Autodesk Inventor part; units mm, degrees
ref_plane "Start Plane" through (0, 0, -2.9702) normal (0, 0, 1) x (1, 0, 0)
ref_plane "End Plane" through (0, 0, 105) normal (0, 0, 1) x (1, 0, 0)
ref_plane "Work Plane4" through (0, -10, -2.9702) normal (0, 0.2847, -0.9586) x (1, 0, 0)
ref_plane "Start Plane" through (0, 0, -2.9702) normal (0, 0, 1) x (1, 0, 0)
ref_plane "End Plane" through (0, 0, 105) normal (0, 0, 1) x (1, 0, 0)
sketch "Sketch" plane through (0, 0, 0) normal (0, 0, 1) x (1, 0, 0)
  line L0 (-10, -7) -> (-10, 7)
  line L1 (-7, 10) -> (7, 10)
  line L2 (10, 7) -> (10, -7)
  line L3 (7, -10) -> (-7, -10)
  arc A0 (-10, -7) -> (-7, -10) centre (-7, -7) ccw
  arc A1 (-7, 10) -> (-10, 7) centre (-7, 7) ccw
  arc A2 (10, 7) -> (7, 10) centre (7, 7) ccw
  arc A3 (7, -10) -> (10, -7) centre (7, -7) ccw
  arc A4 (-7, 8) -> (-8, 7) centre (-7, 7) ccw
  line L4 (-7, 8) -> (7, 8)
  arc A5 (8, 7) -> (7, 8) centre (7, 7) ccw
  line L5 (8, 7) -> (8, -7)
  arc A6 (7, -8) -> (8, -7) centre (7, -7) ccw
  line L6 (7, -8) -> (-7, -8)
  arc A7 (-8, -7) -> (-7, -8) centre (-7, -7) ccw
  line L7 (-8, -7) -> (-8, 7)
  line L8 (0, 14.8698) -> (0, -14.8698) construction
  line L9 (-14.8698, 0) -> (14.8698, 0) construction
  dimension "d7" = 3
  dimension "d10" = 20
  dimension "d11" = 20
  dimension "d12" = 2
  dimension "d15" = 10
  dimension "d16" = 10
extrude "Body" add sketch "Sketch" along normal up to surface (107.9702 mm away) from surface at -2.9702
sketch "Sketch3" plane through (0, 0, 0) normal (0, 0, 1) x (1, 0, 0)
  line L0 (0, 0) -> (10, 0)
ref_plane "Work Plane3" through (0, 0, 0) normal (0, -1, 0) x (1, 0, 0)
sketch "Sketch4" plane through (0, 0, 0) normal (0, -1, 0) x (1, 0, 0)
  line L0 (-2, -2.9702) -> (12, -2.9702)
  line L1 (-2, 105) -> (12, 105)
  dimension "d18" = 107.9702
ref_plane "Work Plane4" through (0, -10, -2.9702) normal (0, 0.2847, -0.9586) x (1, 0, 0)
split "Split1" plane through (0, -10, -2.9702) removes the side toward (0, 0.2847, -0.9586)
sketch "Sketch5" plane through (-7, -10, 105) normal (0, -1, 0) x (1, 0, 0)
  line L0 (0, 0) -> (14, 0)
  line L1 (7, 0) -> (7, -18) construction
  line L2 (13.85, 0) -> (0.15, 0)
  line L3 (0.15, 0) -> (0.15, -18)
  line L4 (0.15, -18) -> (13.85, -18)
  line L5 (13.85, -18) -> (13.85, 0)
  line L6 (14, 0) -> (0, 0)
  line L7 (13.85, -8) -> (0.15, -8)
  line L8 (0.15, -8) -> (0.15, -26)
  line L9 (0.15, -26) -> (13.85, -26)
  line L10 (13.85, -26) -> (13.85, -8)
  line L11 (13.85, -8) -> (0.15, -26) construction
  line L12 (0.15, -8) -> (13.85, -26) construction
  line L13 (13.85, -8) -> (17, -8)
  line L14 (17, 0) -> (17, -102.9209)
  line L15 (17, -8) -> (17, 0)
  line L16 (17, 0) -> (13.85, 0)
  line L17 (-3, 0) -> (0, 0)
  line L18 (0.15, 0) -> (-3, 0)
  line L19 (-3, 0) -> (-3, -8)
  line L20 (-3, -8) -> (0.15, -8)
  point P0 (7, -105)
  point P1 (7, 0)
  point P2 (13.85, 0)
  point P3 (0.15, 0)
  point P4 (7, -17)
  point P5 (13.85, -18)
  point P6 (0.15, -18)
  point P7 (13.85, -8)
  point P8 (17, -8)
  point P9 (0.15, -8)
  dimension "d19" = 13.7
  dimension "d20" = 18
  dimension "d23" = 13.7
  dimension "d24" = 18
  dimension "d25" = 8
extrude "Extrusion2" cut sketch "Sketch5" against normal through all
equation "\"d7\" = G_IR"
equation "\"d10\" = G_H"
equation "\"d11\" = G_W"
equation "\"d12\" = G_T"
equation "\"d15\" = 0.5 * d10"
equation "\"d16\" = 0.5 * d11"
equation "\"d3\" = G_L"
equation "\"d23\" = d19"
equation "\"d24\" = d20"
equation "\"G_W\" = 20"
equation "\"G_H\" = 20"
equation "\"G_T\" = 2"
equation "\"G_IR\" = 3"
equation "\"G_L\" = d18"
equation "\"G_OFFSET_START\" = 2.97016"
equation "\"G_OFFSET_END\" = 0"
equation "\"d13\" = -G_OFFSET_START"
equation "\"d14\" = G_OFFSET_END + B_L"
equation "\"B_L\" = 105"
properties part number "ISO 12633-2 - 20x20x2 - 107,97" material "Steel, Mild"
Work out the finished part from the listing and answer in its coordinate system (mm). A direction names the side the tool comes from. Round coordinates to 2 decimals unless told otherwise and drop trailing zeros. Order: outer loops, then holes, each group sorted by start corner. A loop starts at its lowest first (then second) coordinate and runs counter-clockwise, first axis right, second up.
Q1. Given pin 1 Ø0.6 at (x, y) = (-2.5, -9.5) entering from +Z; pin 2 Ø12 at (x, y) = (-7, -6) entering from +Z; pin 3 Ø0.6 at (y, z) = (9, 89) entering from -X; pin 4 Ø1 at (y, z) = (9.5, 91.5) entering from +X, each flat-ended and moving along its own axis, determine where each tip first touches the part or whether it passes through.
Solution:
pin 1: stops at z = 79
pin 2: stops at z = 97
pin 3: stops at x = -9.47
pin 4: stops at x = 9.24
Q2. A tool of negligible diameter and unlimited length cuts with its end or side. For faces 1 (the flat face through (0, -8, 36)), 2 (the flat face through (-6.85, -9, 88)), 3 (the flat face through (0, -10, 35)), from which of +Z, -Z, +X, -X, +Y, -Y can it reach the whole face along a straight path? Write none if from no direction.
Solution:
face 1: +Z, -Z
face 2: +Z, +Y, -Y
face 3: +Z, -Z, +X, -X, -Y
Q3. Find the intervals of material crossed by line 1 along Y through (x, z) = (-3.25, 74); line 2 along X through (y, z) = (-7.5, 40), in increasing order.
Solution:
line 1: y = -10 to -8, 8 to 10
line 2: x = -9.96 to -7.87, 7.87 to 9.96
Q4. A cutting plane is placed at B-B, the plane z = 87. Determine the outline of the cut face in (x, y), then the cut area to 3 significant figures.
Solution:
outline: (-10, -7) arc R3 ccw to (-7, -10) - (-6.85, -10) - (-6.85, -8) - (-7, -8) arc R1 cw to (-8, -7) - (-8, 7) arc R1 cw to (-7, 8) - (-6.85, 8) - (-6.85, 10) - (-7, 10) arc R3 ccw to (-10, 7) - close; (6.85, -10) - (7, -10) arc R3 ccw to (10, -7) - (10, 7) arc R3 ccw to (7, 10) - (6.85, 10) - (6.85, 8) - (7, 8) arc R1 cw to (8, 7) - (8, -7) arc R1 cw to (7, -8) - (6.85, -8) - close
area: 82.3 mm2
Q5. The mould has two halves that part along X. Classify faces 4 (the cylindrical face through (-9.1, -9.14, 46.32)), 5 (the cylindrical face through (9.14, -9.1, 46.32)), 6 (the flat face through (0, 9, 79)), 7 (the flat face through (-8, 0, 47)): pulls with the +X half, pulls with the -X half, needs draft (parallel to the pull), parting line crosses it, or undercut.
Solution:
face 4: pulls with the -X half
face 5: pulls with the +X half
face 6: undercut
face 7: undercut
Q6. A cutting plane is placed at D-D, the plane y = 4. Determine the outline of the cut face in (x, z), then the cut area to 3 significant figures.
Solution:
outline: (-10, 1.19) - (-8, 1.19) - (-8, 97) - (-10, 97) - close; (8, 1.19) - (10, 1.19) - (10, 97) - (8, 97) - close
area: 383 mm2
Q7. A cutting plane is placed at A-A, the plane x = -5.25. Determine the outline of the cut face in (y, z).
Solution:
outline: (-10, -2.97) - (-8, -2.38) - (-8, 79) - (-10, 79) - close; (8, 2.38) - (10, 2.97) - (10, 79) - (8, 79) - close
Q8. A cutting plane is placed at C-C, the plane z = 4. Determine the outline of the cut face in (x, y).
Solution:
outline: (-10, -7) arc R3 ccw to (-7, -10) - (7, -10) arc R3 ccw to (10, -7) - (10, 7) arc R3 ccw to (7, 10) - (-7, 10) arc R3 ccw to (-10, 7) - close; hole (-8, -7) arc R1 ccw to (-7, -8) - (7, -8) arc R1 ccw to (8, -7) - (8, 7) arc R1 ccw to (7, 8) - (-7, 8) arc R1 ccw to (-8, 7) - close
